from build123d import *

# Parameters (mm, degrees)
CYLINDER083_R          = 1.6
CYLINDER083_DEPTH      = 10
CYLINDER081_R          = 1.6
CYLINDER081_DEPTH      = 10
CYLINDER082_R          = 1.6
CYLINDER082_DEPTH      = 10
CYLINDER084_R          = 1.6
CYLINDER084_DEPTH      = 10
CYLINDER095_R          = 4
CYLINDER095_DEPTH      = 3
CYLINDER096_R          = 4
CYLINDER096_DEPTH      = 3
CYLINDER097_R          = 4
CYLINDER097_DEPTH      = 3
CYLINDER094_R          = 4
CYLINDER094_DEPTH      = 3
BOX039_W               = 80
BOX039_H               = 5
BOX039_DEPTH           = 50
FILLET028_R            = 3
FILLET029_R            = 3
CUT063_PLACEMENT_ANGLE = 3


with BuildPart() as cylinder083:
    # Cylinder083 → Cylinder083 (new body)
    with BuildSketch(Plane(origin=(76.5, 96, 46.5), x_dir=(1, 0, 0), z_dir=(0, -1, 0))):
        Circle(CYLINDER083_R)
    extrude(amount=CYLINDER083_DEPTH)


with BuildPart() as cylinder081:
    # Cylinder081 → Cylinder081 (new body)
    with BuildSketch(Plane(origin=(76.5, 96, 3.5), x_dir=(1, 0, 0), z_dir=(0, -1, 0))):
        Circle(CYLINDER081_R)
    extrude(amount=CYLINDER081_DEPTH)


with BuildPart() as cylinder082:
    # Cylinder082 → Cylinder082 (new body)
    with BuildSketch(Plane(origin=(3.5, 96, 46.5), x_dir=(1, 0, 0), z_dir=(0, -1, 0))):
        Circle(CYLINDER082_R)
    extrude(amount=CYLINDER082_DEPTH)


with BuildPart() as fusion073:
    # Cylinder084 → Cylinder084 (new body)
    with BuildSketch(Plane(origin=(3.5, 96, 3.5), x_dir=(1, 0, 0), z_dir=(0, -1, 0))):
        Circle(CYLINDER084_R)
    extrude(amount=CYLINDER084_DEPTH)

    # Fusion073: union Cylinder083, Cylinder081, Cylinder082
    add(cylinder083.part)
    add(cylinder081.part)
    add(cylinder082.part)


with BuildPart() as fusion073_1:
    # Fusion073 placement: moved
    add(fusion073.part.moved(Location((0, 5, 0))))


with BuildPart() as cylinder095:
    # Cylinder095 → Cylinder095 (new body)
    with BuildSketch(Plane(origin=(76.5, 96, 46.5), x_dir=(1, 0, 0), z_dir=(0, -1, 0))):
        Circle(CYLINDER095_R)
    extrude(amount=CYLINDER095_DEPTH)


with BuildPart() as cylinder096:
    # Cylinder096 → Cylinder096 (new body)
    with BuildSketch(Plane(origin=(76.5, 96, 3.5), x_dir=(1, 0, 0), z_dir=(0, -1, 0))):
        Circle(CYLINDER096_R)
    extrude(amount=CYLINDER096_DEPTH)


with BuildPart() as cylinder097:
    # Cylinder097 → Cylinder097 (new body)
    with BuildSketch(Plane(origin=(3.5, 96, 46.5), x_dir=(1, 0, 0), z_dir=(0, -1, 0))):
        Circle(CYLINDER097_R)
    extrude(amount=CYLINDER097_DEPTH)


with BuildPart() as fusion082:
    # Cylinder094 → Cylinder094 (new body)
    with BuildSketch(Plane(origin=(3.5, 96, 3.5), x_dir=(1, 0, 0), z_dir=(0, -1, 0))):
        Circle(CYLINDER094_R)
    extrude(amount=CYLINDER094_DEPTH)

    # Fusion082: union Cylinder095, Cylinder096, Cylinder097
    add(cylinder095.part)
    add(cylinder096.part)
    add(cylinder097.part)


with BuildPart() as fusion082_1:
    # Fusion082 placement: moved
    add(fusion082.part.moved(Location((0, 5, 0))))


with BuildPart() as battery_holder_cap:
    # Box039 → Box039 (new body)
    with BuildSketch(Plane(origin=(0, 96, 0), x_dir=(1, 0, 0), z_dir=(0, 0, 1))):
        with Locations((40, 2.5)):
            Rectangle(BOX039_W, BOX039_H)
    extrude(amount=BOX039_DEPTH)

    # Fillet028
    fillet028_edges = [battery_holder_cap.edges().sort_by_distance(p)[0] for p in [
        (0, 98.5, 50),
        (0, 98.5, 0),
        (80, 98.5, 50),
        (80, 98.5, 0),
    ]]
    fillet(fillet028_edges, radius=FILLET028_R)

    # Fillet029
    fillet029_edges = [battery_holder_cap.edges().sort_by_distance(p)[0] for p in [
        (0, 101, 25),
        (40, 101, 0),
        (80, 101, 25),
        (40, 101, 50),
    ]]
    fillet(fillet029_edges, radius=FILLET029_R)

    # Fusion102: union Fusion082
    add(fusion082_1.part)

    # Cut063: cut Fusion073
    add(fusion073_1.part, mode=Mode.SUBTRACT)


with BuildPart() as battery_holder_cap_1:
    # Cut063 placement: moved
    add(battery_holder_cap.part.moved(Location((306, -5, -55))).rotate(Axis((306, -5, -55), (0, -1, 0)), CUT063_PLACEMENT_ANGLE))


solid = battery_holder_cap_1.part
Input: part model. Units: mm. Frame: model coordinates. A direction names the side the tool comes from. Round coordinates to 2 decimals unless told otherwise and drop trailing zeros. Order: outer loops, then holes, each group sorted by start corner. A loop starts at its lowest first (then second) coordinate and runs counter-clockwise, first axis right, second up. Notation, with made-up numbers: (-38, -36.5) - (-30, -36.5) arc R17 ccw to (-30, -6.5) - close; hole circle Ø7 at (53.5, 30.25). An arc over 180 degrees is marked (long way). Answer as a JSON object with one key per item and string values. Group by question number.
(1) Draft query along Z for faces 4 (the face through (381.46, 93.54, -4)), 5 (the face through (345.428, 92.014, -52.934)), 6 (the face through (342.811, 92.014, -3.002)), 7 (the face through (380.612, 93.535, -47.514)). Return one class per face: released by +Z, released by -Z, zero draft, split by the parting line, or undercut.
(2) Reachability of faces 1 (the face through (383.74, 95.1, -26.17)), 2 (the face through (304.174, 94.521, -5.613)), 3 (the face through (343.856, 95.098, -3.804)) from +Z, -Z, +X, -X, +Y, -Y: full face, straight path, thin tool, end or side. Return the list, or none.
(3) Cut plane A-A (y = 94.6). Return loops of the section in (x, z).
(4) Material intervals for probe 1 along X at (y, z) = (91.5, -47.5); probe 2 along Z at (x, y) = (310.5, 92.7); probe 3 along Z at (x, y) = (336.5, 93.1), sorted ascending. Write a range as from..to.
(5) Pin query (flat end, axial travel): P1, Ø1, axis at x = 348, y = 93.5, coming from the -Z side; P2, Ø2, axis at y = 94.5, z = -21, coming from the -X side; P3, Ø1, axis at x = 343, y = 94, coming from the -Z side; P4, Ø3.5, axis at x = 307.06, z = -8.38, coming from the +Y side. Return the tip coordinate at first contact, or that it passes through.
Here are the results:
{
 "1": {"face 4": "undercut", "face 5": "released by -Z", "face 6": "released by +Z", "face 7": "undercut"},
 "2": {"face 1": "+X, +Y", "face 2": "+Y", "face 3": "+Z, +Y"},
 "3": {"outline": "(304.16, -11.14) - (306.14, -48.88) arc R4 ccw to (312.07, -54.22) - (379.77, -50.67) arc R4 ccw to (385.11, -44.74) - (383.13, -7) arc R4 ccw to (377.2, -1.66) - (309.5, -5.21) arc R4 ccw to start; hole circle Ø3.2 at (307.06, -8.38); hole circle Ø3.2 at (309.31, -51.32); hole circle Ø3.2 at (379.96, -4.56); hole circle Ø3.2 at (382.21, -47.5)"},
 "4": {"probe 1": "x = 305.61..380.61, 383.81..385.72", "probe 2": "z = -54.76..-52.39, -50.25..-4.7", "probe 3": "z = -53.4..-3.33"},
 "5": {"P1": "stops at z = -52.81", "P2": "stops at x = 304.25", "P3": "stops at z = -53.02", "P4": "stops at y = 96"}
}
